Can you work these out from the model? Positions are in its coordinate system, mm. A direction names the side the tool comes from. Give positions to 0.01 mm unless a question says otherwise; leave off trailing zeros. Loops run counter-clockwise (first coordinate to the right, second up) from the corner with the lowest first, then second, coordinate; pieces in that order, holes last. Notation, with made-up numbers: M -14,71.25 L -2,71.25 A18 cw -2,79.25 Z; hole C 74.5,35.5 d5. An arc over 180 degrees is marked long. Put each result on its own line as item: value. Start each with the question number.
1) Please list where these lines run through material, in increasing order: line 1 along X through (y, z) = (-7, 4.5); line 2 along X through (y, z) = (-7.5, 31); line 3 along Y through (x, z) = (-3, 49.5). Write a range as from..to.
2) Imagine slicing it at A-A (x = -2.25). Write out the boundary of the cut face in (y, z).
3) For faces 1 (the flat face through (-4, -9, 29)), 2 (the cylindrical face through (-0.1, -12.3, 28.9)), 3 (the flat face through (3, -9, 29)), which set-ups out of +Z, -Z, +X, -X, +Y, -Y let a thin tool reach every point of the face, with its end or its side?
4) For P1, Ø1, axis at x = -2.5, z = 37, coming from the -Y side; P2, Ø1.5, axis at x = 0.5, z = 13.5, coming from the +Y side, each with a flat end and sliding along its axis, tell me the tip position at first contact or that it passes through.
from build123d import *

# Parameters (mm, degrees)
BOX004_W                   = 3.5
BOX004_H                   = 3
BOX004_DEPTH               = 60
BOX003_W                   = 3.5
BOX003_H                   = 3
BOX003_DEPTH               = 60
EXTRUDE009_DEPTH           = 55
EXTRUDE009_PLACEMENT_ANGLE = 180
FILLET004_R                = 2
FILLET005_R                = 1


with BuildPart() as obj1:
    # Box004 → Box004 (new body)
    with BuildSketch(Plane(origin=(1.75, -9, 0), x_dir=(1, 0, 0), z_dir=(0, 0, 1))):
        with Locations((1.75, 1.5)):
            Rectangle(BOX004_W, BOX004_H)
    extrude(amount=BOX004_DEPTH)


with BuildPart() as obj2:
    # Box003 → Box003 (new body)
    with BuildSketch(Plane(origin=(-5.25, -9, 0), x_dir=(1, 0, 0), z_dir=(0, 0, 1))):
        with Locations((1.75, 1.5)):
            Rectangle(BOX003_W, BOX003_H)
    extrude(amount=BOX003_DEPTH)


with BuildPart() as obj3:
    # Sketch007 → Extrude009 (new body)
    with BuildSketch(Plane.XY):
        with BuildLine():
            ThreePointArc((-5.868808, 10.809583), (0, 6.057418), (5.868808, 10.809583))
            ThreePointArc((5.868808, 10.809583), (0, 12.3), (-5.868808, 10.809583))
        make_face()
    extrude(amount=EXTRUDE009_DEPTH)


with BuildPart() as obj3_1:
    # Extrude009 placement: moved
    add(obj3.part.moved(Location((0, 0, 1.8))).rotate(Axis((0, 0, 1.8), (0, 0, 1)), EXTRUDE009_PLACEMENT_ANGLE))

    # Fillet004
    fillet004_edges = [obj3_1.edges().sort_by_distance(p)[0] for p in [
        (5.868808, -10.809583, 29.3),
        (-5.868808, -10.809583, 29.3),
    ]]
    fillet(fillet004_edges, radius=FILLET004_R)

    # Cut002: cut obj2
    add(obj2.part, mode=Mode.SUBTRACT)

    # Cut003: cut obj1
    add(obj1.part, mode=Mode.SUBTRACT)

    # Fillet005
    fillet005_edges = [obj3_1.edges().sort_by_distance(p)[0] for p in [
        (-1.75, -6.318298, 29.3),
        (1.75, -6.318298, 29.3),
        (-1.75, -9, 29.3),
        (1.75, -9, 29.3),
        (5.125721, -9, 29.3),
        (-5.125721, -9, 29.3),
    ]]
    fillet(fillet005_edges, radius=FILLET005_R)


solid = obj3_1.part
Recorded:
1. line 1: -1.74..1.74
1. line 2: -1.75..1.75
1. line 3: -11.93..-9
2. outline: M -12.09,1.8 L -8.87,1.8 L -8.87,56.8 L -12.09,56.8 Z
3. face 1: +Z, -Z, -X, +Y
3. face 2: +Z, -Z, -Y
3. face 3: +Z, -Z, +X, +Y
4. P1: y = -12.14
4. P2: y = -6.06
